The model under review builds one solid part; all positions refer to its coordinate system, in mm. Round coordinates to 2 decimals unless told otherwise and drop trailing zeros. Write each loop counter-clockwise with the first axis right and the second up, starting at its lowest first coordinate (ties: lowest second). Pieces come first, ordered by that corner, then holes. Notation, with made-up numbers: (-16.5, -10.75) - (12.5, -10.75) arc R22 ccw to (12.5, 3.25) - close; hole circle Ø11 at (-9.5, 15.5). An arc over 180 degrees is marked (long way). Write each question's results on one line, items separated by ' | '.
```python
from build123d import *

# Parameters (mm, degrees)
SKETCH1_R      = 4.7625
SKETCH1_R_2    = 3.175
EXTRUDE1_DEPTH = 6.35
SKETCH3_R      = 4.7625
SKETCH3_R_2    = 3.175
SKETCH5_R      = 4.7625
SKETCH5_R_2    = 3.175


with BuildPart() as part:
    # Sketch1 → Extrude1 (new, symmetric)
    with BuildSketch(Plane(origin=(0, 0, 0), x_dir=(0, 0, -1), z_dir=(1, 0, 0))):
        Circle(SKETCH1_R)
        Circle(SKETCH1_R_2, mode=Mode.SUBTRACT)
    extrude(amount=EXTRUDE1_DEPTH, both=True)

    # Sweep1: sweep along a path in Sketch6
    with BuildLine(Plane.XY) as sweep1_path:
        ThreePointArc((-6.35, 0), (-56.222049707, -11.726919872), (-95.642120974, -44.45))
    # Sketch3 → Sweep1 (sweep)
    with BuildSketch(Plane.ZY.offset(6.35)):
        Circle(SKETCH3_R)
        Circle(SKETCH3_R_2, mode=Mode.SUBTRACT)
    sweep(path=sweep1_path.line)

    # Sweep2: sweep along a path in Sketch4
    with BuildLine(Plane.XY) as sweep2_path:
        ThreePointArc((95.642120974, -44.45), (56.222049707, -11.726919872), (6.35, 0))
    # Sketch5 → Sweep2 (sweep)
    with BuildSketch(Plane(origin=(6.35, 0, 0), x_dir=(0, 0, -1), z_dir=(1, 0, 0))):
        Circle(SKETCH5_R)
        Circle(SKETCH5_R_2, mode=Mode.SUBTRACT)
    sweep(path=sweep2_path.line)


solid = part.part
```
Q1. For probe 1 along Y at (x, z) = (3.25, 0) (1 decimal); probe 2 along X at (y, z) = (-31, -2.5); probe 3 along X at (y, z) = (-23.5, 0.5), list the stretches that pass through material, from the lowest coordinate up.
Evaluation:
probe 1: y = -4.8 to -3.2, 3.2 to 4.8 | probe 2: x = -89.42 to -86.47, -80.8 to -77.67, 77.67 to 80.8, 86.47 to 89.42 | probe 3: x = -82.44 to -79.96, -69.72 to -66.93, 66.93 to 69.72, 79.96 to 82.44
Q2. We need section A-A (z = 0.5). State the section outline as (x, y) points, plus the area to 3 significant figures.
Evaluation:
outline: (-99.42, -41.59) - (-98.14, -42.56) arc R115.05 cw to (-6.35, 3.14) - (6.35, 3.14) arc R115.05 cw to (98.14, -42.56) - (99.42, -41.59) arc R116.65 ccw to (6.35, 4.74) - (-6.35, 4.74) arc R116.65 ccw to start; (-93.14, -46.34) - (-91.86, -47.31) arc R107.17 cw to (-6.35, -4.74) - (6.35, -4.74) arc R107.17 cw to (91.86, -47.31) - (93.14, -46.34) arc R108.78 ccw to (6.35, -3.14) - (-6.35, -3.14) arc R108.78 ccw to start | area: 703 mm^2
Q3. The part is to be moulded in two halves that separate along Z. For faces 1 (the cylindrical face through (0.09, -2.9, 3.78)), 2 (the cylindrical face through (-0.09, -3.1, 0.69)), say which applies: released by +Z, released by -Z, zero draft, split by the parting line, or undercut.
Evaluation:
face 1: split by the parting line | face 2: undercut
Q4. We need section C-C (y = -18.5). State how many separate pieces and enclosed holes the cut face has, plus the area to 3 significant figures.
Evaluation:
separate pieces: 2 | enclosed holes: 2 | area: 145 mm^2
Q5. Insertion check: P1, Ø1.5, axis at x = -30, z = 3, coming from the +Y side; P2, Ø3, axis at x = 70.5, y = -16.5, coming from the +Z side; P3, Ø1.5, axis at y = -24, z = -3.5, coming from the -X side. Each pin has a flat end and moves straight along its axis. Give the tip position at first contact, or say it passes through.
Evaluation:
P1: stops at y = 1.79 | P2: stops at z = 4.5 | P3: stops at x = -82.09
